Source: CAD feature listing. Evaluate the final solid. Frame: model axes, mm. Face numbers are marked on the shaded views. Round coordinates to 2 decimals unless told otherwise and drop trailing zeros. Loops run counter-clockwise (first coordinate to the right, second up) from the corner with the lowest first, then second, coordinate; pieces in that order, holes last. Notation, with made-up numbers: (50.25, 53.25) -> (67.25, 53.25) arc R32 ccw to (67.25, 87.25) -> close; hole circle Ø11 at (-11, -6). An arc over 180 degrees is marked (long way). Return JSON: item names as keys, results as strings. Group by question number.
Autodesk Inventor part; units mm, degrees
ref_plane "YZ Plane" through (0, 0, 0) normal (1, 0, 0) x (0, 1, 0)
ref_plane "XZ Plane" through (0, 0, 0) normal (0, 1, 0) x (-1, 0, 0)
ref_plane "XY Plane" through (0, 0, 0) normal (0, 0, 1) x (1, 0, 0)
ref_plane "Work Plane1" through (-10, 7, -20) normal (0, 1, 0) x (1, 0, 0)
sketch "Sketch3" plane through (-10, 7, -20) normal (0, 1, 0) x (1, 0, 0)
  circle A0 centre (5.4301, -4.6077) radius 2 construction
  line L0 (4.1095, -3.1058) -> (5.5583, -2.6118)
  line L1 (5.5583, -2.6118) -> (6.9321, -3.287)
  line L2 (6.9321, -3.287) -> (7.426, -4.7359)
  line L3 (7.426, -4.7359) -> (6.7508, -6.1096)
  line L4 (6.7508, -6.1096) -> (5.302, -6.6036)
  line L5 (5.302, -6.6036) -> (3.9282, -5.9284)
  line L6 (3.9282, -5.9284) -> (3.4343, -4.4795)
  line L7 (3.4343, -4.4795) -> (4.1095, -3.1058)
  point P0 (10, -20)
extrude "Extrusion1" add sketch "Sketch3" along normal blind 10
chamfer "Chamfer1" distance 0.5 angle 45 8 edges at (-3.9736, 7, -13.6434) (-2.9116, 7, -14.5772) (-2.8209, 7, -15.9886) (-3.7548, 7, -17.0506) (-5.1661, 7, -17.1412) (-6.2281, 7, -16.2073) (-6.3188, 7, -14.796) (-5.3849, 7, -13.734)
chamfer "Chamfer2" distance 0.5 angle 45 8 edges at (-5.3849, 17, -13.734) (-3.9736, 17, -13.6434) (-6.3188, 17, -14.796) (-6.2281, 17, -16.2073) (-5.1661, 17, -17.1412) (-3.7548, 17, -17.0506) (-2.8209, 17, -15.9886) (-2.9116, 17, -14.5772)
sketch "Sketch4" plane through (-10, 17, -20) normal (0, 1, 0) x (1, 0, 0)
  line L0 (5.5236, -3.1519) -> (6.5257, -3.6444) construction
  line L1 (4.4668, -3.5122) -> (5.5236, -3.1519) construction
  line L2 (3.9743, -4.5142) -> (4.4668, -3.5122) construction
  line L3 (4.3346, -5.571) -> (3.9743, -4.5142) construction
  line L4 (5.3367, -6.0635) -> (4.3346, -5.571) construction
  line L5 (6.3935, -5.7032) -> (5.3367, -6.0635) construction
  line L6 (6.886, -4.7012) -> (6.3935, -5.7032) construction
  line L7 (6.5257, -3.6444) -> (6.886, -4.7012) construction
  point P0 (10, -20)
  point P1 (5.4301, -4.6077)
hole "Hole1" at (-4.5699, 17, -15.3923) direction (0, -1, 0) diameter 2.5 end through all
properties part number "pin_oct_4mm"
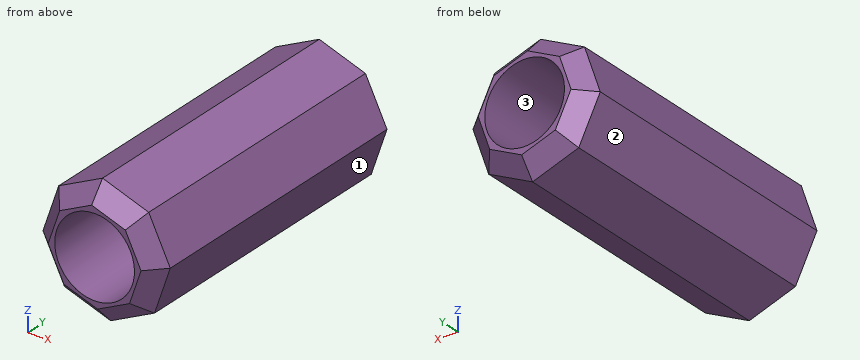
(1) Mould query, pull axis X, two halves, no side actions, for the marked faces 1, 2 and 3. Classes: released by +X, released by -X, zero draft, split by the parting line, or undercut.
(2) Cut plane A-A (x = -5.25). Return loops of the section in (y, z), and give its area (3 significant figures).
(3) Ray query, line 1 (Z direction, x = -5.55, y = 9.5); line 2 (X direction, y = 11.5, z = -15.65); line 3 (X direction, y = 10.25, z = -14.4). Return the intervals inside material, ascending.
(4) Cut plane D-D (x = -6.25). Return loops of the section in (y, z).
(5) Cut plane B-B (z = -14.6). Return loops of the section in (x, y), and give its area (3 significant figures).
(6) Cut plane C-C (y = 10.25). Return loops of the section in (x, z), and give its area (3 significant figures).
(7) Pin query (flat end, axial travel): pin 1 (1.5 mm diameter, centred on x = -4.57, z = -15.39, fed in from -Y); pin 2 (1.5 mm diameter, centred on y = 11.5, z = -14.5, fed in from -X). Return the tip coordinate at first contact, or that it passes through.
Answers follow:
{
 "1": {"face 1": "released by +X", "face 2": "released by -X", "face 3": "undercut"},
 "2": {"outline": "(7, -16.58) -> (7.5, -17.11) -> (16.5, -17.11) -> (17, -16.58) -> (17, -16.44) -> (7, -16.44) -> close; (7, -14.34) -> (17, -14.34) -> (17, -14.22) -> (16.5, -13.67) -> (7.5, -13.67) -> (7, -14.22) -> close", "area": "12.9 mm^2"},
 "3": {"line 1": "-17.01 to -16.17, -14.62 to -13.82", "line 2": "-6.5 to -5.79, -3.35 to -2.71", "line 3": "-6.18 to -5.33, -3.81 to -3"},
 "4": {"outline": "(7.21, -15.5) -> (7.5, -16.16) -> (16.5, -16.16) -> (16.79, -15.5) -> (16.5, -14.59) -> (7.5, -14.59) -> close"},
 "5": {"outline": "(-6.25, 7.5) -> (-5.72, 7) -> (-5.54, 7) -> (-5.54, 17) -> (-5.72, 17) -> (-6.25, 16.5) -> close; (-3.6, 7) -> (-3.46, 7) -> (-2.9, 7.5) -> (-2.9, 16.5) -> (-3.46, 17) -> (-3.6, 17) -> close", "area": "13.6 mm^2"},
 "6": {"outline": "(-6.57, -15.52) -> (-5.89, -16.89) -> (-4.44, -17.39) -> (-3.07, -16.71) -> (-2.57, -15.26) -> (-3.25, -13.89) -> (-4.7, -13.4) -> (-6.07, -14.07) -> close; hole circle Ø2.5 at (-4.57, -15.39)", "area": "6.40 mm^2"},
 "7": {"pin 1": "through", "pin 2": "x = -6.47"}
}
